Work out the finished part from the listing and answer in its coordinate system (mm). Coordinates: 2 decimals unless noted, no trailing zeros. Order: outer loops, then holes, each group sorted by start corner. A loop starts at its lowest first (then second) coordinate and runs counter-clockwise, first axis right, second up. Notation, with made-up numbers: (50.25, 27.25) -> (71.25, 27.25) arc R16 ccw to (71.25, 37.25) -> close; hole circle Ø6 at (-33.5, -22.5). An arc over 180 degrees is marked (long way). Use one line per item in the form item = value.
Autodesk Inventor part; units mm, degrees
ref_plane "YZ Plane" through (0, 0, 0) normal (1, 0, 0) x (0, 1, 0)
ref_plane "XZ Plane" through (0, 0, 0) normal (0, 1, 0) x (-1, 0, 0)
ref_plane "XY Plane" through (0, 0, 0) normal (0, 0, 1) x (1, 0, 0)
sketch "Szkic1" plane through (0, 0, 0) normal (0, 0, 1) x (1, 0, 0)
  line L0 (500, -450) -> (-500, -450)
  line L1 (-500, -450) -> (-500, 450)
  line L2 (-500, 450) -> (500, 450)
  line L3 (500, 450) -> (500, -450)
  line L4 (500, -450) -> (-500, 450) construction
  line L5 (-500, -450) -> (500, 450) construction
  circle A0 centre (250, -200) radius 75
  line L6 (505, -455) -> (-505, -455) construction
  line L7 (-505, -455) -> (-505, 455) construction
  line L8 (-505, 455) -> (505, 455) construction
  line L9 (505, 455) -> (505, -455) construction
  line L10 (505, -455) -> (-505, 455) construction
  line L11 (-505, -455) -> (505, 455) construction
  line L12 (480, -430) -> (-480, -430) construction
  line L13 (-480, -430) -> (-480, 430) construction
  line L14 (-480, 430) -> (480, 430) construction
  line L15 (480, 430) -> (480, -430) construction
  line L16 (480, -430) -> (-480, 430) construction
  line L17 (-480, -430) -> (480, 430) construction
  circle A1 centre (-470, 0) radius 3
  circle A2 centre (-470, 350) radius 3
  circle A3 centre (-470, -350) radius 3
  circle A4 centre (-470, 0) radius 3
  line L18 (0, -722.0928) -> (0, 703.6821)
  line L19 (480, -430) -> (480, 430) construction
  circle A5 centre (470, 350) radius 3
  circle A6 centre (470, -350) radius 3
  circle A7 centre (470, 0) radius 3
  circle A8 centre (0, 420) radius 3
  circle A9 centre (380, 420) radius 3
  circle A10 centre (-380, 420) radius 3
  circle A11 centre (0, 420) radius 3
  line L20 (-763, 0) -> (763, 0)
  circle A12 centre (0, -420) radius 3
  circle A13 centre (380, -420) radius 3
  circle A14 centre (-380, -420) radius 3
  line L21 (545, -500) -> (-545, -500) construction
  line L22 (-545, -500) -> (-545, 500) construction
  line L23 (-545, 500) -> (545, 500) construction
  line L24 (545, 500) -> (545, -500) construction
  line L25 (545, -500) -> (-545, 500) construction
  line L26 (-545, -500) -> (545, 500) construction
  line L27 (-372.8845, -485.3907) -> (-256.6542, -485.3907) construction
  line L28 (-256.6542, -485.3907) -> (-256.6542, -518.4107) construction
  line L29 (-256.6542, -518.4107) -> (-372.8845, -518.4107) construction
  line L30 (-372.8845, -518.4107) -> (-372.8845, -485.3907) construction
  point P0 (0, 0)
  dimension "d0" = 1000
  dimension "d1" = 900
  dimension "d2" = 150
  dimension "d3" = 250
  dimension "d4" = 250
  dimension "d5" = 1010
  dimension "d6" = 910
  dimension "d7" = 25
  dimension "d8" = 25
  dimension "d9" = 6
  dimension "d10" = 10
  dimension "d13" = 350
  dimension "d16" = 350
  dimension "d19" = 6
  dimension "d20" = 10
  dimension "d23" = 380
  dimension "d26" = 380
  dimension "d31" = 1090
  dimension "d32" = 1000
extrude "Wyciągnięcie proste1" add sketch "Szkic1" along normal blind 3 contours L0 L18 A12 L20 A7 L3 | L0 L1 L20 A1 L18 A12 | L20 A7 L18 A8 L2 L3 | L1 L2 L18 A8 L20 A1
properties part number "PLEXI 1"
(1) Straight lines are drawn through the part: line 1 along Y through (x, z) = (0, 0.95); line 2 along Y through (x, z) = (470, 1.25); line 3 along X through (y, z) = (420, 0.9). For each, find the intervals that lie inside material, in ascending order.
Data:
line_1 = -450 to -423, -417 to 417, 423 to 450
line_2 = -450 to -353, -347 to -3, 3 to 347, 353 to 450
line_3 = -500 to -383, -377 to -3, 3 to 377, 383 to 500
(2) Section B-B on z = 2.5 is taken. Count the separate pieces of the cut face and the enclosed holes in it, plus the area to 3 significant figures.
Data:
separate_pieces = 1
enclosed_holes = 13
area = 882,000 mm²
(3) The mould has two halves that part along Y. Classify faces 1 (the cylindrical face through (290.32, -263.24, 1.48)), 2 (the flat face through (-7, 6, 3)): released by +Y, released by -Y, zero draft, split by the parting line, or undercut.
Data:
face_1 = undercut
face_2 = zero draft
(4) Section A-A on y = -200 is taken. Write down the section's boundary in (x, z).
Data:
outline = (-500, 0) -> (175, 0) -> (175, 3) -> (-500, 3) -> close; (325, 0) -> (500, 0) -> (500, 3) -> (325, 3) -> close
